```python
from build123d import *

# Parameters (mm, degrees)
SKETCH1_R                    = 20
BOSS_EXTRUDE1_DEPTH          = 15
SKETCH4_R                    = 14.5
CUT_EXTRUDE3_DEPTH           = 12
SKETCH5_R                    = 10.5
CUT_EXTRUDE4_DEPTH           = 12
SKETCH6_R                    = 1.5
CUT_EXTRUDE5_DEPTH           = 33.015621187
SKETCH7_R                    = 2.5
CUT_EXTRUDE7_DEPTH           = 2
CUT_EXTRUDE7_DRAFT           = -27
CUT_EXTRUDE7_PROFILE_2_DEPTH = 2
CUT_EXTRUDE7_PROFILE_2_DRAFT = -27
CUT_EXTRUDE7_PROFILE_3_DEPTH = 2
CUT_EXTRUDE7_PROFILE_3_DRAFT = -27
CUT_EXTRUDE7_PROFILE_4_DEPTH = 2
CUT_EXTRUDE7_PROFILE_4_DRAFT = -27


with BuildPart() as part:
    # Sketch1 → Boss-Extrude1 (new body)
    with BuildSketch(Plane(origin=(0, 0, 0), x_dir=(1, 0, 0), z_dir=(0, 1, 0))):
        with Locations(Location((0, 0, 0), (0, 0, 270))):
            Circle(SKETCH1_R)
    extrude(amount=BOSS_EXTRUDE1_DEPTH)

    # Sketch4 → Cut-Extrude3 (cut)
    with BuildSketch(Plane.XZ):
        with Locations(Location((0, 0, 0), (0, 0, 270))):
            Circle(SKETCH4_R)
    extrude(amount=-CUT_EXTRUDE3_DEPTH, mode=Mode.SUBTRACT)

    # Sketch5 → Cut-Extrude4 (cut)
    with BuildSketch(Plane(origin=(0, 15, 0), x_dir=(1, 0, 0), z_dir=(0, 1, 0))):
        with Locations(Location((0, 0, 0), (0, 0, 270))):
            Circle(SKETCH5_R)
    extrude(amount=-CUT_EXTRUDE4_DEPTH, mode=Mode.SUBTRACT)

    # Sketch6 → Cut-Extrude5 (cut, through all)
    with BuildSketch(Plane(origin=(0, 15, 0), x_dir=(1, 0, 0), z_dir=(0, 1, 0))):
        with Locations(Location((0, 17, 0), (0, 0, 270))):
            Circle(SKETCH6_R)
        with Locations(Location((17, 0, 0), (0, 0, 270))):
            Circle(SKETCH6_R)
        with Locations(Location((0, -17, 0), (0, 0, 270))):
            Circle(SKETCH6_R)
        with Locations(Location((-17, 0, 0), (0, 0, 270))):
            Circle(SKETCH6_R)
    extrude(amount=-CUT_EXTRUDE5_DEPTH, mode=Mode.SUBTRACT)


with BuildPart() as cut_extrude7_tool:
    # Sketch7 → Cut-Extrude7 (with draft: the straight prism first)
    with BuildSketch(Plane(origin=(0, 15, 0), x_dir=(1, 0, 0), z_dir=(0, 1, 0))):
        with Locations((0, 17)):
            Circle(SKETCH7_R)
    extrude(amount=-CUT_EXTRUDE7_DEPTH)
    # Cut-Extrude7: the draft: its side faces are tilted about the plane it starts from
    cut_extrude7_sides = [cut_extrude7_tool.faces().sort_by_distance(p)[0] for p in [
        (-2.5, 14, -17),
    ]]
    draft(cut_extrude7_sides, Plane(origin=(0, 15, 0), x_dir=(1, 0, 0), z_dir=(0, 1, 0)), CUT_EXTRUDE7_DRAFT)


with BuildPart() as part_1:
    add(part.part)

    # Cut-Extrude7: cut by cut_extrude7_tool
    add(cut_extrude7_tool.part, mode=Mode.SUBTRACT)


with BuildPart() as cut_extrude7_profile_2_tool:
    # Sketch7 → Cut-Extrude7 profile 2 (with draft: the straight prism first)
    with BuildSketch(Plane(origin=(0, 15, 0), x_dir=(1, 0, 0), z_dir=(0, 1, 0))):
        with Locations((17, 0)):
            Circle(SKETCH7_R)
    extrude(amount=-CUT_EXTRUDE7_PROFILE_2_DEPTH)
    # Cut-Extrude7 profile 2: the draft: its side faces are tilted about the plane it starts from
    cut_extrude7_profile_2_sides = [cut_extrude7_profile_2_tool.faces().sort_by_distance(p)[0] for p in [
        (14.5, 14, 0),
    ]]
    draft(cut_extrude7_profile_2_sides, Plane(origin=(0, 15, 0), x_dir=(1, 0, 0), z_dir=(0, 1, 0)), CUT_EXTRUDE7_PROFILE_2_DRAFT)


with BuildPart() as part_2:
    add(part_1.part)

    # Cut-Extrude7 profile 2: cut by cut_extrude7_profile_2_tool
    add(cut_extrude7_profile_2_tool.part, mode=Mode.SUBTRACT)


with BuildPart() as cut_extrude7_profile_3_tool:
    # Sketch7 → Cut-Extrude7 profile 3 (with draft: the straight prism first)
    with BuildSketch(Plane(origin=(0, 15, 0), x_dir=(1, 0, 0), z_dir=(0, 1, 0))):
        with Locations((0, -17)):
            Circle(SKETCH7_R)
    extrude(amount=-CUT_EXTRUDE7_PROFILE_3_DEPTH)
    # Cut-Extrude7 profile 3: the draft: its side faces are tilted about the plane it starts from
    cut_extrude7_profile_3_sides = [cut_extrude7_profile_3_tool.faces().sort_by_distance(p)[0] for p in [
        (-2.5, 14, 17),
    ]]
    draft(cut_extrude7_profile_3_sides, Plane(origin=(0, 15, 0), x_dir=(1, 0, 0), z_dir=(0, 1, 0)), CUT_EXTRUDE7_PROFILE_3_DRAFT)


with BuildPart() as part_3:
    add(part_2.part)

    # Cut-Extrude7 profile 3: cut by cut_extrude7_profile_3_tool
    add(cut_extrude7_profile_3_tool.part, mode=Mode.SUBTRACT)


with BuildPart() as cut_extrude7_profile_4_tool:
    # Sketch7 → Cut-Extrude7 profile 4 (with draft: the straight prism first)
    with BuildSketch(Plane(origin=(0, 15, 0), x_dir=(1, 0, 0), z_dir=(0, 1, 0))):
        with Locations((-17, 0)):
            Circle(SKETCH7_R)
    extrude(amount=-CUT_EXTRUDE7_PROFILE_4_DEPTH)
    # Cut-Extrude7 profile 4: the draft: its side faces are tilted about the plane it starts from
    cut_extrude7_profile_4_sides = [cut_extrude7_profile_4_tool.faces().sort_by_distance(p)[0] for p in [
        (-19.5, 14, 0),
    ]]
    draft(cut_extrude7_profile_4_sides, Plane(origin=(0, 15, 0), x_dir=(1, 0, 0), z_dir=(0, 1, 0)), CUT_EXTRUDE7_PROFILE_4_DRAFT)


with BuildPart() as part_4:
    add(part_3.part)

    # Cut-Extrude7 profile 4: cut by cut_extrude7_profile_4_tool
    add(cut_extrude7_profile_4_tool.part, mode=Mode.SUBTRACT)


solid = part_4.part
```
Geometry check sheet. Reference: the model listing, model coordinates, mm. A direction names the side the tool comes from. Coordinates: 2 decimals unless noted, no trailing zeros. Order: outer loops, then holes, each group sorted by start corner. A loop starts at its lowest first (then second) coordinate and runs counter-clockwise, first axis right, second up. Notation, with made-up numbers: (32.5, 31.5) - (68.5, 31.5) arc R13 ccw to (68.5, 40.5) - close; hole circle Ø9 at (1, 7.5). An arc over 180 degrees is marked (long way). Answer as a JSON object with one key per item and string values. Group by question number.
Item 1: Tool access check on faces 4 (the face through (-5.554, 5.916, -13.394)), 5 (the face through (-15.513, 6.61, -0.195)). Record the directions out of +Z, -Z, +X, -X, +Y, -Y that give a thin tool (end or side, any length) a straight path to the whole face; none if there is none.
Item 2: Sectioned sample at D-D, the plane z = 17. Record the cut outline in (x, y).
Item 3: Sectioned sample at A-A, the plane z = 0. Record the cut outline in (x, y).
Item 4: Sectioned sample at B-B, the plane x = -7. Record the cut outline in (y, z) (3 decimals), and give its area (3 significant figures).
Item 5: Scan lines: probe 1 along X at (y, z) = (7.25, 0); probe 2 along X at (y, z) = (10, -17); probe 3 along X at (y, z) = (2.25, 6.5). Record each from-to range of solid material in increasing order.
Item 6: Sectioned sample at C-C, the plane y = 3.5. Record the cut outline in (x, z), and give its area (3 significant figures).
Item 7: Depth check by flat-ended pin: pin 1 Ø3 at (x, y) = (11, 7.5) entering from -Z; pin 2 Ø3 at (x, y) = (14.5, 12) entering from -Z; pin 3 Ø6 at (y, z) = (9, -11.5) entering from +X; pin 4 Ø2.5 at (x, z) = (0, -17) entering from +Y. Enter the tip coordinate at first touch or a pass-through.
Item 8: Draft check along X on faces 1 (the face through (-19.524, 7.395, -4.336)), 2 (the face through (1.5, 13.2, 16.5)), 3 (the face through (-9, 15, 9)). Enter one of: +X half, -X half, draft (parallel to the pull), parting line (faces both ways), or undercut.
Resolved:
{
 "1": {"face 4": "-Y", "face 5": "+Y, -Y"},
 "2": {"outline": "(-10.54, 0) - (-1.5, 0) - (-1.5, 13.04) - (-2.5, 15) - (-10.54, 15) - close; (1.5, 0) - (10.54, 0) - (10.54, 15) - (2.5, 15) - (1.5, 13.04) - close"},
 "3": {"outline": "(-20, 0) - (-18.5, 0) - (-18.5, 13.04) - (-19.5, 15) - (-20, 15) - close; (-15.5, 0) - (-14.5, 0) - (-14.5, 12) - (-10.5, 12) - (-10.5, 15) - (-14.5, 15) - (-15.5, 13.04) - close; (10.5, 12) - (14.5, 12) - (14.5, 0) - (15.5, 0) - (15.5, 13.04) - (14.5, 15) - (10.5, 15) - close; (18.5, 0) - (20, 0) - (20, 15) - (19.5, 15) - (18.5, 13.04) - close"},
 "4": {"outline": "(0, -18.735) - (15, -18.735) - (15, -7.826) - (12, -7.826) - (12, -12.698) - (0, -12.698) - close; (0, 12.698) - (12, 12.698) - (12, 7.826) - (15, 7.826) - (15, 18.735) - (0, 18.735) - close", "area": "210 mm^2"},
 "5": {"probe 1": "-20 to -18.5, -15.5 to -14.5, 14.5 to 15.5, 18.5 to 20", "probe 2": "-10.54 to -1.5, 1.5 to 10.54", "probe 3": "-18.91 to -12.96, 12.96 to 18.91"},
 "6": {"outline": "circle Ø40 at (0, 0); hole circle Ø3 at (-17, 0); hole circle Ø29 at (0, 0); hole circle Ø3 at (0, -17); hole circle Ø3 at (0, 17); hole circle Ø3 at (17, 0)", "area": "568 mm^2"},
 "7": {"pin 1": "z = -17.6", "pin 2": "z = -15.2", "pin 3": "x = 18.1", "pin 4": "through"},
 "8": {"face 1": "parting line", "face 2": "undercut", "face 3": "draft"}
}
